```python
from build123d import *

# Parameters (mm, degrees)
SKETCH1_W            = 40
SKETCH1_H            = 20
BOSS_EXTRUDE1_DEPTH  = 15
SHELL2_T             = -2
CUT_EXTRUDE1_START   = -11
CUT_EXTRUDE1_DEPTH   = 2.5
MIRROR2_START        = -11
MIRROR2_COPY_1_DEPTH = 2.5


with BuildPart() as part:
    # Sketch1 → Boss-Extrude1 (new body)
    with BuildSketch(Plane(origin=(0, 0, 0), x_dir=(1, 0, 0), z_dir=(0, 1, 0))):
        Rectangle(SKETCH1_W, SKETCH1_H)
    extrude(amount=BOSS_EXTRUDE1_DEPTH)

    # Shell2
    shell2_openings = [part.faces().sort_by_distance(p)[0] for p in [
        (0, 15, 0),
    ]]
    offset(amount=SHELL2_T, openings=shell2_openings, kind=Kind.INTERSECTION)

    # Sketch2 → Cut-Extrude1 (cut, symmetric)
    with BuildSketch(Plane(origin=(0, 0, 0), x_dir=(0, 0, -1), z_dir=(1, 0, 0)).offset(CUT_EXTRUDE1_START)):
        with BuildLine():
            Line((8.25, 15), (8.25, 12.144151844))
            ThreePointArc((8.25, 12.144151844), (8.287751563, 12.027209787), (8.386754447, 11.954415184))
            Line((8.386754447, 11.954415184), (9, 11.75))
            Line((9, 11.75), (8.25, 10))
            Line((8.25, 10), (7.25, 10))
            Line((7.25, 10), (7.25, 15))
            Line((7.25, 15), (8.25, 15))
        make_face()
    cut_extrude1 = extrude(amount=CUT_EXTRUDE1_DEPTH, both=True, mode=Mode.SUBTRACT)

    # Mirror1: Cut-Extrude1 across plane
    add(cut_extrude1.mirror(Plane(origin=(0, 0, 0), x_dir=(0, 0, 1), z_dir=(1, 0, 0))), mode=Mode.SUBTRACT)

    # Mirror2: Cut-Extrude1 across plane
    add(cut_extrude1.mirror(Plane.XY), mode=Mode.SUBTRACT)

    # Mirror2 copy 1 sketch → Mirror2 copy 1 (cut, symmetric)
    with BuildSketch(Plane.ZY.offset(MIRROR2_START)):
        with BuildLine():
            Line((8.25, 15), (8.25, 12.144151844))
            ThreePointArc((8.25, 12.144151844), (8.287751563, 12.027209787), (8.386754447, 11.954415184))
            Line((8.386754447, 11.954415184), (9, 11.75))
            Line((9, 11.75), (8.25, 10))
            Line((8.25, 10), (7.25, 10))
            Line((7.25, 10), (7.25, 15))
            Line((7.25, 15), (8.25, 15))
        make_face()
    extrude(amount=MIRROR2_COPY_1_DEPTH, both=True, mode=Mode.SUBTRACT)


solid = part.part
```
Geometry: final body of the model. Coordinates: model frame, mm. A direction names the side the tool comes from. Round coordinates to 2 decimals unless told otherwise and drop trailing zeros. Loops run counter-clockwise (first coordinate to the right, second up) from the corner with the lowest first, then second, coordinate; pieces in that order, holes last.
Item 1: Line query: L1, parallel to X at y = 6.5, z = 6.75; L2, parallel to Z at x = 1, y = 3; L3, parallel to Z at x = -10, y = 14.75. Output: solid intervals per line, ascending.
Checked values:
L1: x = -20 to -18, 18 to 20
L2: z = -10 to -8, 8 to 10
L3: z = -10 to -8.25, 8.25 to 10
Item 2: Reachability of faces 4 (the flat face through (-20, 7, 0)), 5 (the flat face through (8.5, 11.4, -8.3)), 6 (the flat face through (-18, 8, 0)) from +Z, -Z, +X, -X, +Y, -Y: full face, straight path, thin tool, end or side. Return the list, or none.
Checked values:
face 4: +Z, -Z, -X, +Y, -Y
face 5: none
face 6: +Y
Item 3: Section A-A, the plane y = 5. Output: boundary loops of the cut face in (x, z).
Checked values:
outline: (-20, -10) - (20, -10) - (20, 10) - (-20, 10) - close; hole (-18, -8) - (18, -8) - (18, 8) - (-18, 8) - close
Item 4: Contact query for a flat-ended pin moving along its axis: P1, Ø1.5, axis at x = 10.5, z = 4, coming from the +Y side. Output: stop coordinate, or through.
Checked values:
P1: stops at y = 2
Item 5: Section B-B, the plane x = 10. Output: boundary loops of the cut face in (y, z), plus the area to 3 significant figures.
Checked values:
outline: (0, -10) - (15, -10) - (15, -8.25) - (12.14, -8.25) arc R0.2 ccw to (11.95, -8.39) - (11.75, -9) - (10, -8.25) - (10, -8) - (2, -8) - (2, 8) - (10, 8) - (10, 8.25) - (11.75, 9) - (11.95, 8.39) arc R0.2 ccw to (12.14, 8.25) - (15, 8.25) - (15, 10) - (0, 10) - close
area: 88.0 mm2
Item 6: Mould query, pull axis Y, two halves, no side actions, for faces 1 (the flat face through (0, 0, 0)), 2 (the flat face through (0, 7, 10)), 3 (the flat face through (-10.96, 10.89, -8.63)). Classes: released by +Y, released by -Y, zero draft, split by the parting line, or undercut.
Checked values:
face 1: released by -Y
face 2: zero draft
face 3: undercut
Item 7: Section D-D, the plane x = 16. Output: boundary loops of the cut face in (y, z).
Checked values:
outline: (0, -10) - (15, -10) - (15, -8) - (2, -8) - (2, 8) - (15, 8) - (15, 10) - (0, 10) - close
Item 8: Section C-C, the plane z = -1.75. Output: boundary loops of the cut face in (x, y).
Checked values:
outline: (-20, 0) - (20, 0) - (20, 15) - (18, 15) - (18, 2) - (-18, 2) - (-18, 15) - (-20, 15) - close
